Autodesk Inventor part; units mm, degrees
ref_plane "YZ Plane" through (0, 0, 0) normal (1, 0, 0) x (0, 1, 0)
ref_plane "XZ Plane" through (0, 0, 0) normal (0, 1, 0) x (-1, 0, 0)
ref_plane "XY Plane" through (0, 0, 0) normal (0, 0, 1) x (1, 0, 0)
sketch "Sketch1" plane through (0, 0, 0) normal (0, 0, 1) x (1, 0, 0)
  circle A0 centre (0, 0) radius 4.572
  dimension "d0" = 9.144
extrude "Extrusion1" add sketch "Sketch1" along normal blind 2.54
fillet "Fillet1" radius 0.635 1 edges at (-4.572, 0, 2.54)
sketch "Sketch2" plane through (0, 0, 2.54) normal (0, 0, 1) x (1, 0, 0)
  line L0 (-0.5978, 1.4024) -> (2.1711, 1.4024) construction
  line L1 (2.1711, 1.4024) -> (2.1711, -1.6456) construction
  line L2 (2.1711, -1.6456) -> (-0.5978, -1.6456) construction
  line L3 (-0.5978, -1.6456) -> (-0.5978, 1.4024) construction
  line L4 (-0.4421, -1.6456) -> (-0.4421, 1.4024)
  line L5 (-0.4421, 1.4024) -> (0.1271, 1.4024)
  spline S0 degree 2 poles (0.1271, 1.4024) (0.3013, 1.4024) (0.5127, 1.2166) (0.6312, 0.8332) (0.6312, 0.6218) knots 0 0 0 1 2 3 3 3
  spline S1 degree 2 poles (0.6312, 0.6218) (0.6312, 0.4267) (0.5267, 0.0829) (0.4198, -0.024) knots 0 0 0 1 2 2 2
  spline S2 degree 2 poles (0.4198, -0.024) (0.5569, -0.1053) (0.7055, -0.4956) (0.7055, -0.7628) knots 0 0 0 1 2 2 2
  spline S3 degree 2 poles (0.7055, -0.7628) (0.7055, -0.9765) (0.6149, -1.3436) (0.4825, -1.5434) (0.2827, -1.6456) (0.1364, -1.6456) knots 0 0 0 1 2 3 4 4 4
  line L6 (0.1364, -1.6456) -> (-0.4421, -1.6456)
  line L7 (-0.24, -1.2855) -> (0.1387, -1.2855)
  spline S4 degree 2 poles (0.1387, -1.2855) (0.2363, -1.2855) (0.2758, -1.2716) knots 0 0 0 1 1 1
  spline S5 degree 2 poles (0.2758, -1.2716) (0.3455, -1.246) (0.4384, -1.1298) (0.4988, -0.9068) (0.4988, -0.7605) knots 0 0 0 1 2 3 3 3
  spline S6 degree 2 poles (0.4988, -0.7605) (0.4988, -0.5909) (0.4105, -0.34) (0.2549, -0.2377) (0.1108, -0.2377) knots 0 0 0 1 2 3 3 3
  line L8 (0.1108, -0.2377) -> (-0.24, -0.2377)
  line L9 (-0.24, -0.2377) -> (-0.24, -1.2855)
  line L10 (-0.24, 0.1224) -> (0.0876, 0.1224)
  spline S7 degree 2 poles (0.0876, 0.1224) (0.2223, 0.1224) (0.2804, 0.1572) knots 0 0 0 1 1 1
  spline S8 degree 2 poles (0.2804, 0.1572) (0.3571, 0.2037) (0.4337, 0.4151) (0.4337, 0.5754) knots 0 0 0 1 2 2 2
  spline S9 degree 2 poles (0.4337, 0.5754) (0.4337, 0.7264) (0.3617, 0.9564) (0.227, 1.0423) (0.0644, 1.0423) knots 0 0 0 1 2 3 3 3
  line L11 (0.0644, 1.0423) -> (-0.24, 1.0423)
  line L12 (-0.24, 1.0423) -> (-0.24, 0.1224)
extrude "Extrusion2" cut sketch "Sketch2" against normal blind 0.0635
properties part number "B Button"
Check sheet for the modelled part. Datum: model origin and axes. Units: mm. Give positions to 0.01 mm unless a question says otherwise; leave off trailing zeros. Write each loop counter-clockwise with the first axis right and the second up, starting at its lowest first coordinate (ties: lowest second). Pieces come first, ordered by that corner, then holes.
Item 1: Scan lines: L1, parallel to Z at x = 3.75, y = 2.5 (3 decimals); L2, parallel to Y at x = 3, z = 1.4; L3, parallel to Y at x = -2.75, z = 1.85. Record each from-to range of solid material in increasing order.
Item 2: Cross-section at A-A (z = 1.15). Enter the section's corners in (x, y).
Item 3: Gauge pin test, flat ends, axial feed: pin 1 (4 mm diameter, centred on x = -2, y = -2.5, fed in from -Z); pin 2 (1.5 mm diameter, centred on x = -2, z = 1, fed in from -Y). Record the tip position at first contact, or that the pin passes through.
Item 4: Cross-section at B-B (z = 2.2). Enter the section's corners in (x, y), and give its area (3 significant figures).
Report:
1. L1: z = 0 to 2.185
1. L2: y = -3.45 to 3.45
1. L3: y = -3.65 to 3.65
2. outline: circle Ø9.14 at (0, 0)
3. pin 1: stops at z = 0
3. pin 2: stops at y = -4.4
4. outline: circle Ø9 at (0, 0)
4. area: 63.6 mm2
